Build history of the part. All positions in model axes, mm. A direction names the side the tool comes from. Round coordinates to 2 decimals unless told otherwise and drop trailing zeros. Loops run counter-clockwise (first coordinate to the right, second up) from the corner with the lowest first, then second, coordinate; pieces in that order, holes last. Notation, with made-up numbers: (72, 60.25) - (78, 60.25) arc R5 cw to (78, 66.25) - close; hole circle Ø9 at (-14, 4). An arc over 180 degrees is marked (long way). Put each result on its own line as item: value. Start each with the question number.
from build123d import *

# Parameters (mm, degrees)
CROQUIS1_W              = 33
CROQUIS1_H              = 15
CROQUIS1_W_2            = 30
CROQUIS1_H_2            = 12
SALIENTE_EXTRUIR1_DEPTH = 9
CROQUIS2_W              = 33
CROQUIS2_H              = 15
SALIENTE_EXTRUIR2_DEPTH = 1.5
CROQUIS3_R              = 1
CORTAR_EXTRUIR1_DEPTH   = 1.5


with BuildPart() as part:
    # Croquis1 → Saliente-Extruir1 (new body)
    with BuildSketch(Plane.XY):
        with Locations((-37.090098455, 21.435354346)):
            Rectangle(CROQUIS1_W, CROQUIS1_H)
        with Locations((-37.090098455, 21.435354346)):
            Rectangle(CROQUIS1_W_2, CROQUIS1_H_2, mode=Mode.SUBTRACT)
    extrude(amount=SALIENTE_EXTRUIR1_DEPTH)

    # Croquis2 → Saliente-Extruir2 (add)
    with BuildSketch(Plane.XY):
        with Locations((-37.090098455, 21.435354346)):
            Rectangle(CROQUIS2_W, CROQUIS2_H)
    extrude(amount=-SALIENTE_EXTRUIR2_DEPTH)

    # Croquis3 → Cortar-Extruir1 (cut)
    with BuildSketch(Plane.XY):
        with Locations((-37.090098455, 21.435354346)):
            Circle(CROQUIS3_R)
    extrude(amount=-CORTAR_EXTRUIR1_DEPTH, mode=Mode.SUBTRACT)


solid = part.part
Item 1: Slice it at D-D (x = -40.5). Give the cut face in (y, z).
Item 2: Slice it at B-B (y = 25.5). Give the cut face in (x, z), plus the area to 3 significant figures.
Item 3: Which spindle directions (+Z, -Z, +X, -X, +Y, -Y) get a long thin tool onto all of the face, cutting with end or side? Do faces 4 (the flat face through (-37, 20, 0)), 5 (the flat face through (-37, 23, -1.5)). Say none if no direction does.
Item 4: Two-plate mould, pull along Y, no slides. Class faces 1 (the flat face through (-52.09, 21, 4)), 2 (the flat face through (-38, 15, 9)), 3 (the flat face through (-37, 28.935, 4)): pulls with the +Y half, pulls with the -Y half, needs draft (parallel to the pull), parting line crosses it, or undercut.
Item 5: Drop a flat-ended pin along its axis: pin 1 Ø2.5 at (x, y) = (-37.09, 21.44) entering from +Z. Give the stop position or say it passes through.
Item 6: Drill centre lines: probe 1 along X at (y, z) = (22.75, 3.75); probe 2 along Y at (x, z) = (-32.5, 8.5); probe 3 along Z at (x, y) = (-38, 23). Where is each one in solid material? Low to high. Write a range as [from, to].
Item 7: Slice it at C-C (y = 22). Give the cut face in (x, z), plus the area to 3 significant figures.
Item 8: Slice it at A-A (z = 2). Give the cut face in (x, y), plus the area to 3 significant figures.
Computed values:
1. outline: (13.94, -1.5) - (28.94, -1.5) - (28.94, 9) - (27.44, 9) - (27.44, 0) - (15.44, 0) - (15.44, 9) - (13.94, 9) - close
2. outline: (-53.59, -1.5) - (-20.59, -1.5) - (-20.59, 9) - (-22.09, 9) - (-22.09, 0) - (-52.09, 0) - (-52.09, 9) - (-53.59, 9) - close
2. area: 76.5 mm^2
3. face 4: +Z
3. face 5: -Z, +X, -X, +Y, -Y
4. face 1: undercut
4. face 2: needs draft
4. face 3: pulls with the +Y half
5. pin 1: stops at z = 0
6. probe 1: x = [-53.59, -52.09], [-22.09, -20.59]
6. probe 2: y = [13.94, 15.44], [27.44, 28.94]
6. probe 3: z = [-1.5, 0]
7. outline: (-53.59, -1.5) - (-37.92, -1.5) - (-37.92, 0) - (-52.09, 0) - (-52.09, 9) - (-53.59, 9) - close; (-36.26, -1.5) - (-20.59, -1.5) - (-20.59, 9) - (-22.09, 9) - (-22.09, 0) - (-36.26, 0) - close
7. area: 74.0 mm^2
8. outline: (-53.59, 13.94) - (-20.59, 13.94) - (-20.59, 28.94) - (-53.59, 28.94) - close; hole (-52.09, 15.44) - (-22.09, 15.44) - (-22.09, 27.44) - (-52.09, 27.44) - close
8. area: 135 mm^2
